The drawing under review shows one solid part. Ordinate dimensions are in mm from its lowest x, y, z. Round coordinates to 2 decimals unless told otherwise and drop trailing zeros. Write each loop counter-clockwise with the first axis right and the second up, starting at its lowest first coordinate (ties: lowest second). Pieces come first, ordered by that corner, then holes. Notation, with made-up numbers: (43, 50) -> (82, 50) arc R21 cw to (82, 59) -> close; hole circle Ø7 at (38, 4.5). An arc over 180 degrees is marked (long way). Write item = value, one per line. Start each with the question number.
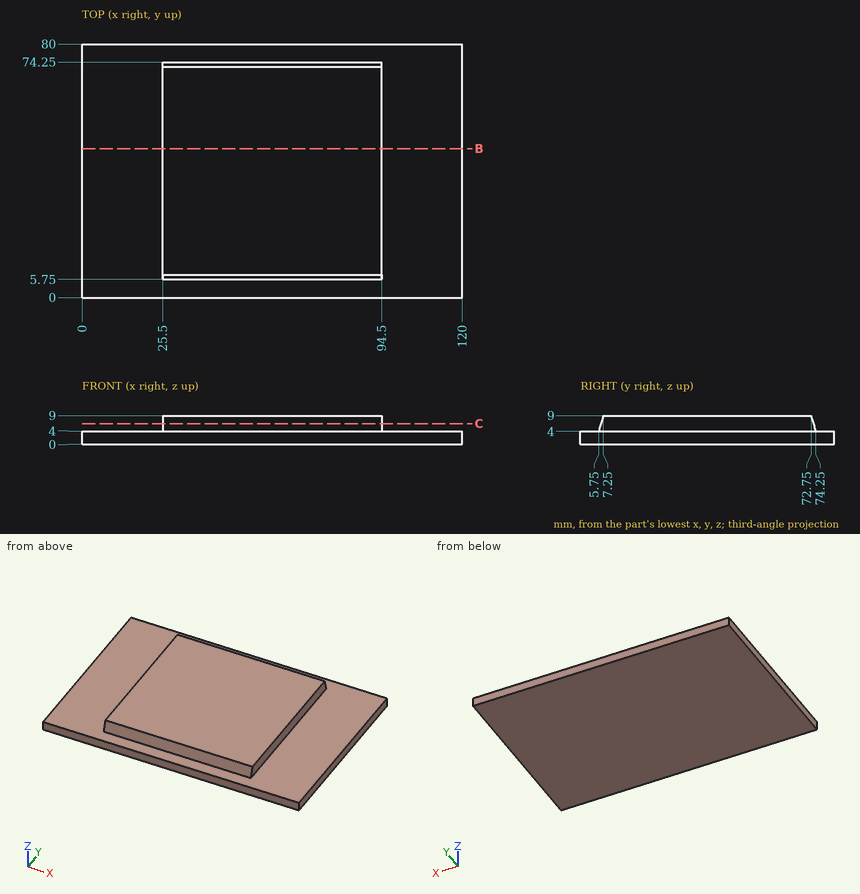
1. Clearance check with flat-ended pins moving along their axes: pin 1 Ø5 at (y, z) = (40, 8) entering from -X; pin 2 Ø4 at (y, z) = (36.5, 7.5) entering from +X. State where each tip first meets the part, or that it passes through.
2. Consider section B-B, the plane y = 47. Give the boundary of the cut face in (x, z).
3. Consider section C-C, the plane z = 6.5. Give the boundary of the cut face in (x, y).
4. Wall thickness on L1, parallel to Z at x = 10, y = 56; L2, parallel to X at y = 50.5, z = 4.5; L3, parallel to Y at x = 62, z = 5.5: over which ranges is each line inside the solid? List them lowest first. Write a range as from..to.
Outcome:
q1.pin_1 = 25.5
q1.pin_2 = 94.5
q2.outline = (0, 0) -> (120, 0) -> (120, 4) -> (94.5, 4) -> (94.5, 9) -> (25.5, 9) -> (25.5, 4) -> (0, 4) -> close
q3.outline = (25.5, 6.5) -> (94.5, 6.5) -> (94.5, 73.5) -> (25.5, 73.5) -> close
q4.L1 = 0..4
q4.L2 = 25.5..94.5
q4.L3 = 6.2..73.8
